```python
from build123d import *

# Parameters (mm, degrees)
SKETCH1_W              = 8
SKETCH1_H              = 5
SKETCH1_W_2            = 10
SKETCH1_H_2            = 8.5
M4_TAPPED_HOLE1_REACH  = 43.337
M4_TAPPED_HOLE1_BORE_R = 1.65


with BuildPart() as part:
    # Sketch1 → Revolve1 (revolve)
    with BuildSketch(Plane.XY, mode=Mode.PRIVATE) as revolve1_sk:
        Polygon((-6.5, 9), (-6.5, 4), (6.5, 4), (6.5, 9), (5, 9), (-5, 9), align=None)
        with Locations((10.5, 6.5)):
            Rectangle(SKETCH1_W, SKETCH1_H)
        with Locations((0, 13.25)):
            Rectangle(SKETCH1_W_2, SKETCH1_H_2)
        Polygon((-6.5, 17.5), (-5, 17.5), (5, 17.5), (6.5, 17.5), (6.5, 22.5), (-6.5, 22.5), align=None)
    revolve(revolve1_sk.sketch.rotate(Axis((0, 0, 0), (1, 0, 0)), 90), axis=Axis((0, 0, 0), (1, 0, 0)))

    # M4 Tapped Hole1 bore → M4 Tapped Hole1 (cut, up to next)
    with BuildSketch(Plane(origin=(0, 9, 0), x_dir=(1, 0, 0), z_dir=(0, 1, 0)), mode=Mode.PRIVATE) as m4_tapped_hole1_sk1:
        with Locations((10.5, 0)):
            Circle(M4_TAPPED_HOLE1_BORE_R)
    m4_tapped_hole1_tool1 = extrude(m4_tapped_hole1_sk1.sketch, amount=-M4_TAPPED_HOLE1_REACH, mode=Mode.PRIVATE) & part.part
    add(m4_tapped_hole1_tool1.solids().sort_by_distance((10.5, 9, 0))[0], mode=Mode.SUBTRACT)


solid = part.part
```
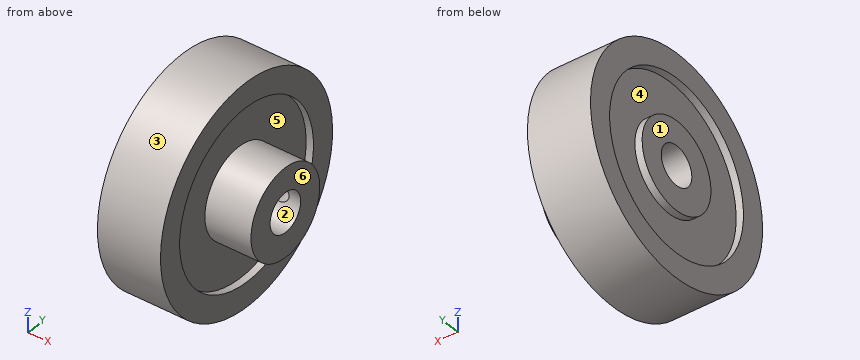
Input: part model. Units: mm. Frame: model coordinates. Face numbers are marked on the shaded views. A direction names the side the tool comes from. Round coordinates to 2 decimals unless told otherwise and drop trailing zeros. Loops run counter-clockwise (first coordinate to the right, second up) from the corner with the lowest first, then second, coordinate; pieces in that order, holes last.
1) Pin query (flat end, axial travel): pin 1 (17.5 mm diameter, centred on y = 7, z = -6, fed in from -X); pin 2 (1.5 mm diameter, centred on x = 11, y = -5.5, fed in from +Z); pin 3 (1 mm diameter, centred on x = 8.5, y = -4.5, fed in from +Z); pin 4 (6 mm diameter, centred on x = 11, y = -1, fed in from +Z). Return the tip coordinate at first contact, or that it passes through.
Ans:
pin 1: stops at x = -6.5
pin 2: stops at z = 7.64
pin 3: stops at z = 8.06
pin 4: stops at z = 9
2) Pull-direction query (Z, two-part tool) for the marked faces 1, 2 and 3; classes: released by +Z, released by -Z, zero draft, split by the parting line, or undercut.
Ans:
face 1: zero draft
face 2: undercut
face 3: split by the parting line
3) Section query A-A on z = 0. Return the cut outline in (x, y).
Ans:
outline: (-6.5, -22.5) - (6.5, -22.5) - (6.5, -17.5) - (5, -17.5) - (5, -9) - (14.5, -9) - (14.5, -4) - (-6.5, -4) - (-6.5, -9) - (-5, -9) - (-5, -17.5) - (-6.5, -17.5) - close; (-6.5, 4) - (8.85, 4) - (8.85, 9) - (5, 9) - (5, 17.5) - (6.5, 17.5) - (6.5, 22.5) - (-6.5, 22.5) - (-6.5, 17.5) - (-5, 17.5) - (-5, 9) - (-6.5, 9) - close; (12.15, 4) - (14.5, 4) - (14.5, 9) - (12.15, 9) - close
4) Section query C-C on x = -2.5. Return the cut outline in (y, z), plus the area to 3 significant figures.
Ans:
outline: circle Ø45 at (0, 0); hole circle Ø8 at (0, 0)
area: 1,540 mm2
5) Section query B-B on y = 0. Return the cut outline in (x, z).
Ans:
outline: (-6.5, -22.5) - (6.5, -22.5) - (6.5, -17.5) - (5, -17.5) - (5, -9) - (14.5, -9) - (14.5, -4) - (-6.5, -4) - (-6.5, -9) - (-5, -9) - (-5, -17.5) - (-6.5, -17.5) - close; (-6.5, 4) - (14.5, 4) - (14.5, 9) - (5, 9) - (5, 17.5) - (6.5, 17.5) - (6.5, 22.5) - (-6.5, 22.5) - (-6.5, 17.5) - (-5, 17.5) - (-5, 9) - (-6.5, 9) - close
6) Set-up query: the marked faces 4, 5 and 6. Return all of +Z, -Z, +X, -X, +Y, -Y with unobstructed straight access to the full face (end or side cutting, diameter ignored); none if empty.
Ans:
face 4: -X
face 5: +X
face 6: +Z, -Z, +X, +Y, -Y
7) Section query D-D on y = 13. Return the cut outline in (x, z), plus the area to 3 significant figures.
Ans:
outline: (-6.5, -18.36) - (6.5, -18.36) - (6.5, -11.72) - (5, -11.72) - (5, 11.72) - (6.5, 11.72) - (6.5, 18.36) - (-6.5, 18.36) - (-6.5, 11.72) - (-5, 11.72) - (-5, -11.72) - (-6.5, -11.72) - close
area: 407 mm2
8) Material intervals for line 1 (X direction, y = 5, z = 0); line 2 (Y direction, x = 9.25, z = 0); line 3 (X direction, y = 11, z = 19), sorted ascending.
Ans:
line 1: x = -6.5 to 8.85, 12.15 to 14.5
line 2: y = -9 to -4
line 3: x = -6.5 to 6.5
